Autodesk Inventor part; units mm, degrees
ref_plane "YZ Plane" through (0, 0, 0) normal (1, 0, 0) x (0, 1, 0)
ref_plane "XZ Plane" through (0, 0, 0) normal (0, 1, 0) x (-1, 0, 0)
ref_plane "XY Plane" through (0, 0, 0) normal (0, 0, 1) x (1, 0, 0)
sketch "スケッチ1" plane through (0, 0, 0) normal (0, 0, 1) x (1, 0, 0)
  line L0 (0, 0) -> (8, 0)
  line L1 (8, 0) -> (8, 1.5)
  line L2 (8, 1.5) -> (0, 1.5)
  line L3 (0, 1.5) -> (0, 0)
  line L4 (0, 0) -> (0, 2.75)
  line L5 (0, 0) -> (-3, 0)
  line L6 (-3, 0) -> (0, 0)
  line L7 (-3, 0) -> (-3, 1.15)
  line L8 (0, 0) -> (-3, 0)
  line L9 (-3, 0) -> (-3, 2.75)
  line L10 (-3, 2.75) -> (0, 2.75)
  line L11 (0, 2.75) -> (0, 0)
  dimension "d0" = 1.5
  dimension "d1" = 8
  dimension "d3" = 3
  dimension "d4" = 2.75
  dimension "d5" = 1.15
revolve "回転1" add sketch "スケッチ1" angle 360 about axis through (-3, 0, 0) along (1, 0, 0)
thread "ねじ1"
sketch "スケッチ2" plane through (-3, 0, 0) normal (-1, 0, 0) x (0, 0, 1)
  circle A0 centre (0, 0) radius 1.15
  line L0 (-0.575, 0.9959) -> (0.575, 0.9959)
  line L1 (0.575, 0.9959) -> (1.15, 0)
  line L2 (1.15, 0) -> (0.575, -0.9959)
  line L3 (0.575, -0.9959) -> (-0.575, -0.9959)
  line L4 (-0.575, -0.9959) -> (-1.15, 0)
  line L5 (-1.15, 0) -> (-0.575, 0.9959)
  dimension "d10" = 1.15
  dimension "d11" = 1.9919
extrude "押し出し1" cut sketch "スケッチ2" against normal blind 1.4 contours L2 L3 L4 L5 L0 L1
fillet "フィレット1" radius 0.2 8 edges at (-1.6, 0.9959, 0) (-1.6, 0.498, 0.8625) (-1.6, 0.498, -0.8625) (-1.6, -0.498, -0.8625) (-1.6, -0.9959, 0) (-1.6, -0.498, 0.8625) (-3, -2.75, 0) (0, -2.75, 0)
fillet "フィレット2" radius 0.1 1 edges at (0, -1.5, 0)
fillet "フィレット3" radius 0.1 1 edges at (8, -1.5, 0)
properties part number "ネジアルミM3L8" material "アルミニウム 7075"
Design review of the part built by this model. Coordinates are the model's own, in mm. A direction names the side the tool comes from. Round coordinates to 2 decimals unless told otherwise and drop trailing zeros. Loops run counter-clockwise (first coordinate to the right, second up) from the corner with the lowest first, then second, coordinate; pieces in that order, holes last. Notation, with made-up numbers: M -5.75,39 L 34.25,39 A19 cw 34.25,58 Z; hole C 55,3.5 d3. An arc over 180 degrees is marked long. Answer as a JSON object with one key per item and string values.
Item 1: We need section A-A on z = 0. Give the boundary of the cut face in (x, y).
Answer sheet:
{"outline": "M -3,-2.55 A0.2 ccw -2.8,-2.75 L -0.2,-2.75 A0.2 ccw 0,-2.55 L 0,-1.6 A0.1 cw 0.1,-1.5 L 7.9,-1.5 A0.1 ccw 8,-1.4 L 8,1.4 A0.1 ccw 7.9,1.5 L 0.1,1.5 A0.1 cw 0,1.6 L 0,2.55 A0.2 ccw -0.2,2.75 L -2.8,2.75 A0.2 ccw -3,2.55 L -3,1 L -1.8,1 A0.2 cw -1.6,0.8 L -1.6,-0.8 A0.2 cw -1.8,-1 L -3,-1 Z"}
Item 2: Clearance check with flat-ended pins moving along their axes: P1, Ø1, axis at x = 6, y = 0.5, coming from the -Z side; P2, Ø2, axis at x = -1.5, z = -1.5, coming from the +Y side; P3, Ø0.5, axis at y = 0, z = -0.5, coming from the -X side. State where each tip first meets the part, or that it passes through.
Answer sheet:
{"P1": "stops at z = -1.5", "P2": "stops at y = 2.7", "P3": "stops at x = -1.6"}
Item 3: Wall thickness on L1, parallel to X at y = -0.7, z = 0.5; L2, parallel to X at y = -1.6, z = 1.9; L3, parallel to Z at x = -2.25, y = 0.55: over which ranges is each line inside the solid? List them lowest first. Write a range as from..to.
Answer sheet:
{"L1": "x = -1.6..8", "L2": "x = -3..0", "L3": "z = -2.69..-0.83, 0.83..2.69"}
Item 4: The part is to be moulded in two halves that separate along Z. For faces 4 (the cylindrical face through (-1.482, -0.596, -2.685)), 5 (the flat face through (-2.41, -0.5, -0.86)), 6 (the flat face through (8, 0, 0)), say which applies: pulls with the +Z half, pulls with the -Z half, needs draft (parallel to the pull), parting line crosses it, or undercut.
Answer sheet:
{"face 4": "parting line crosses it", "face 5": "undercut", "face 6": "needs draft"}
Item 5: We need section B-B on x = 7. Give the boundary of the cut face in (y, z), and give its area (3 significant figures).
Answer sheet:
{"outline": "C 0,0 d3", "area": "7.07 mm^2"}
Item 6: Machinability: for faces 1 (the flat face through (-2.408, 0.491, -0.867)), 2 (the flat face through (-3, 1, -1)), 3 (the flat face through (0, 2, 0)), which of the approach directions +Z, -Z, +X, -X, +Y, -Y give a long, thin tool a straight path to every point of the face, cutting with its end or side? Answer none if there is none.
Answer sheet:
{"face 1": "-X", "face 2": "+Z, -Z, -X, +Y, -Y", "face 3": "+X"}
